from build123d import *

# Parameters (mm, degrees)
SKETCH_1_W          = 27.5
SKETCH_1_H          = 8
EXTRUDE_1_DEPTH     = 5
SKETCH_2_W          = 27.5
SKETCH_2_H          = 2
EXTRUDE_2_DEPTH     = 3
SKETCH_3_R          = 1.5
CUT_EXTRUDE_1_DEPTH = 30.07318352
SKETCH_4_R          = 2.95
CUT_EXTRUDE_6_DEPTH = 3.5
FILLET_1_R          = 1
FILLET_2_R          = 1


with BuildPart() as part:
    # Эскиз1 → Бобышка-Вытянуть1 (new body)
    with BuildSketch(Plane(origin=(0, 0, 0), x_dir=(1, 0, 0), z_dir=(0, 1, 0))):
        with Locations((13.75, 4)):
            Rectangle(SKETCH_1_W, SKETCH_1_H)
    extrude(amount=EXTRUDE_1_DEPTH)

    # Эскиз2 → Бобышка-Вытянуть2 (add)
    with BuildSketch(Plane(origin=(0, 5, 0), x_dir=(1, 0, 0), z_dir=(0, 1, 0))):
        with Locations((13.75, 7)):
            Rectangle(SKETCH_2_W, SKETCH_2_H)
    extrude(amount=EXTRUDE_2_DEPTH)

    # Эскиз3 → Вырез-Вытянуть1 (cut, through all)
    with BuildSketch(Plane(origin=(0, 5, 0), x_dir=(1, 0, 0), z_dir=(0, 1, 0))):
        with Locations(Location((4.5, 3, 0), (0, 0, 270))):
            Circle(SKETCH_3_R)
        with Locations(Location((23, 3, 0), (0, 0, 270))):
            Circle(SKETCH_3_R)
    extrude(amount=-CUT_EXTRUDE_1_DEPTH, mode=Mode.SUBTRACT)

    # Эскиз4 → Вырез-Вытянуть6 (cut)
    with BuildSketch(Plane(origin=(0, 0, 0), x_dir=(-1, 0, 0), z_dir=(0, -1, 0))):
        with Locations(Location((-4.5, 3, 0), (0, 0, 90))):
            Circle(SKETCH_4_R)
        with Locations(Location((-23, 3, 0), (0, 0, 90))):
            Circle(SKETCH_4_R)
    extrude(amount=-CUT_EXTRUDE_6_DEPTH, mode=Mode.SUBTRACT)

    # Скругление1
    fillet_1_edges = [part.edges().sort_by_distance(p)[0] for p in [
        (13.75, 8, -6),
    ]]
    fillet(fillet_1_edges, radius=FILLET_1_R)

    # Скругление2
    fillet_2_edges = [part.edges().sort_by_distance(p)[0] for p in [
        (13.75, 5, 0),
    ]]
    fillet(fillet_2_edges, radius=FILLET_2_R)


solid = part.part
Design review of the part built by this model. Coordinates are the model's own, in mm. A direction names the side the tool comes from. Give positions to 0.01 mm unless a question says otherwise; leave off trailing zeros. Loops run counter-clockwise (first coordinate to the right, second up) from the corner with the lowest first, then second, coordinate; pieces in that order, holes last. Notation, with made-up numbers: (27, 1) - (64, 1) arc R21 ccw to (64, 16) - close; hole circle Ø8 at (26, 86). An arc over 180 degrees is marked (long way). Use CSV: the item, a comma, the result in double quotes. Start each with the question number.
1. Add section A-A (z = -3). State the section outline as (x, y) points, plus the area to 3 significant figures.
2. Draft analysis for pull direction X (two halves, no side actions). For faces 1 (the cylindrical face through (25.487, 1.726, -4.586)), 2 (the flat face through (0, 3, -4)), 3 (the flat face through (21.7, 3.5, -4.3)), 4 (the flat face through (14, 6, -6)), state which applies: released by +X, released by -X, zero draft, split by the parting line, or undercut.
3. Add section D-D (x = 14). State the section outline as (y, z) points, plus the area to 3 significant figures.
4. Add section C-C (y = 2). State the section outline as (x, z) points.
5. Wall thickness on L1, parallel to X at y = 3.9, z = -3; L2, parallel to X at y = 1.1, z = -3; L3, parallel to Y at x = 3, z = -1.25: over which ranges is each line inside the solid? List them lowest first.
6. Machinability: for faces 5 (the cylindrical face through (24.265, 4.26, -2.194)), 6 (the cylindrical face through (7.425, 1.726, -2.616)), 7 (the flat face through (14, 5, -4)), which of the approach directions +Z, -Z, +X, -X, +Y, -Y give a long, thin tool a straight path to every point of the face, cutting with its end or side? Answer none if there is none.
7. Insertion check: P1, Ø2, axis at x = 24, z = -3, coming from the +Y side; P2, Ø3, axis at y = 2, z = -1.5, coming from the -X side; P3, Ø1.8, axis at x = 3.5, z = -4, coming from the -Y side; P4, Ø0.6, axis at x = 7, y = 6.5, coming from the +Z side. Each pin has a flat end and moves straight along its axis. Give the tip position at first contact, or say it passes through.
8. Add section B-B (x = 23). State the section outline as (y, z) points, plus the area to 3 significant figures.
Results found:
1,outline,"(0, 0) - (1.55, 0) - (1.55, 3.5) - (3, 3.5) - (3, 5) - (0, 5) - close; (6, 3.5) - (7.45, 3.5) - (7.45, 0) - (20.05, 0) - (20.05, 3.5) - (21.5, 3.5) - (21.5, 5) - (6, 5) - close; (24.5, 3.5) - (25.95, 3.5) - (25.95, 0) - (27.5, 0) - (27.5, 5) - (24.5, 5) - close"
1,area,"87.2 mm²"
2,face 1,"undercut"
2,face 2,"released by -X"
2,face 3,"undercut"
2,face 4,"zero draft"
3,outline,"(0, -8) - (8, -8) - (8, -7) arc R1 ccw to (7, -6) - (5, -6) - (5, -1) arc R1 ccw to (4, 0) - (0, 0) - close"
3,area,"45.6 mm²"
4,outline,"(0, -8) - (27.5, -8) - (27.5, 0) - (0, 0) - close; hole circle Ø5.9 at (4.5, -3); hole circle Ø5.9 at (23, -3)"
5,L1,"x = 0 to 3, 6 to 21.5, 24.5 to 27.5"
5,L2,"x = 0 to 1.55, 7.45 to 20.05, 25.95 to 27.5"
5,L3,"y = 3.5 to 5"
6,face 5,"+Y, -Y"
6,face 6,"-Y"
6,face 7,"+Z, +X, -X, +Y"
7,P1,"stops at y = 5"
7,P2,"stops at x = 0"
7,P3,"stops at y = 3.5"
7,P4,"stops at z = -6"
8,outline,"(0, -8) - (8, -8) - (8, -7) arc R1 ccw to (7, -6) - (5, -6) - (5, -4.5) - (3.5, -4.5) - (3.5, -5.95) - (0, -5.95) - close; (0, -0.05) - (3.5, -0.05) - (3.5, -1.5) - (5, -1.5) - (5, -1) arc R1 ccw to (4, 0) - (0, 0) - close"
8,area,"20.4 mm²"
